Verification items for this drawing (mm, ordinates from the low corner). Give positions to 0.01 mm unless a question says otherwise; leave off trailing zeros. Loops run counter-clockwise (first coordinate to the right, second up) from the corner with the lowest first, then second, coordinate; pieces in that order, holes last. Notation, with made-up numbers: M -9.75,-24.75 L 22.25,-24.75 A21 cw 22.25,2.25 Z; hole C 36.25,15 d2. An arc over 180 degrees is marked long. Put each result on its own line as item: value. Start each with the question number.
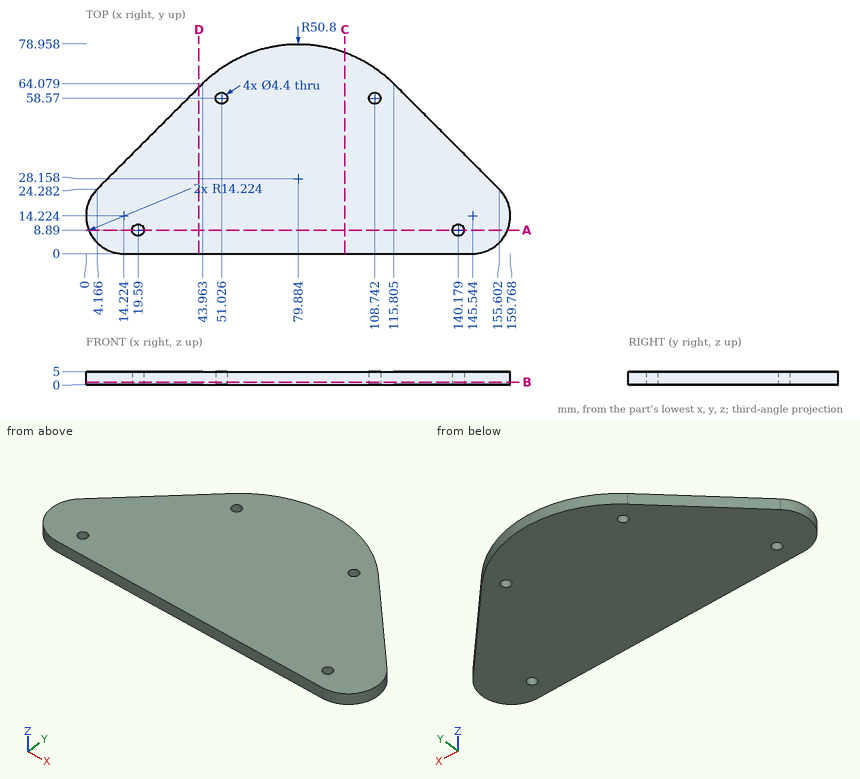
Q1. Cross-section at B-B, the plane z = 1.05. Record the boundary of the cut face in (x, y) (1 decimal).
Q2. Scan lines: L1, parallel to X at y = 9.5, z = 1.6 (1 decimal); L2, parallel to X at y = 60, z = 3.35 (1 decimal); L3, parallel to X at y = 69.5, z = 2.5 (1 decimal). Record each from-to range of solid material in increasing order.
Q3. Go/stop test with a flat-tipped pin: pin 1 (1.5 mm diameter, centred on y = 64.5, z = 2, fed in from +X) (1 decimal). Record where the tip stops, or that it passes through.
Q4. Cross-section at D-D, the plane x = 42.5. Record the boundary of the cut face in (y, z) (1 decimal), then the cut area to 3 significant figures.
Q5. Cross-section at C-C, the plane x = 97.5. Record the boundary of the cut face in (y, z) (1 decimal), then the cut area to 3 significant figures.
Q6. Cross-section at A-A, the plane y = 8.89. Record the boundary of the cut face in (x, z).
Ans:
1. outline: M 4.2,24.3 A14.2 ccw 14.2,0 L 145.5,0 A14.2 ccw 155.6,24.3 L 115.8,64.1 A50.8 ccw 44,64.1 Z; hole C 19.6,8.9 d4.4; hole C 51,58.6 d4.4; hole C 108.7,58.6 d4.4; hole C 140.2,8.9 d4.4
2. L1: x = 0.8 to 17.5, 21.7 to 138.1, 142.3 to 159
2. L2: x = 39.9 to 49.4, 52.7 to 107.1, 110.4 to 119.9
2. L3: x = 50.4 to 109.4
3. pin 1: stops at x = 116.1
4. outline: M 0,0 L 62.6,0 L 62.6,5 L 0,5 Z
4. area: 313 mm^2
5. outline: M 0,0 L 75.8,0 L 75.8,5 L 0,5 Z
5. area: 379 mm^2
6. outline: M 1.04,0 L 17.39,0 L 17.39,5 L 1.04,5 Z; M 21.79,0 L 137.98,0 L 137.98,5 L 21.79,5 Z; M 142.38,0 L 158.73,0 L 158.73,5 L 142.38,5 Z
